Drawing for the job (mm, zero at the part's lowest x, y, z). A direction names the side the tool comes from. Coordinates: 2 decimals unless noted, no trailing zeros. Order: outer loops, then holes, each group sorted by start corner. A loop starts at its lowest first (then second) coordinate and runs counter-clockwise, first axis right, second up.
1) Tool access for the marked faces 1 and 2: list every direction of +Z, -Z, +X, -X, +Y, -Y with a clear straight run to the whole face (end or side of a thin tool).
2) Cut at B-B (z = 39). List the corners of the cut face in (x, y).
3) Pin check, flat tips, straight feed: pin 1 Ø1.5 at (y, z) = (34.5, 56.5) entering from +X; pin 2 Ø2 at (x, y) = (11.5, 38.5) entering from +Z; pin 3 Ø1.5 at (y, z) = (15.5, 17.5) entering from -X. Stop position of each tip, or through.
4) Wall check: L1, parallel to Y at x = 68.5, z = 47.5; L2, parallel to Z at x = 66.5, y = 35.5; L3, parallel to Z at x = 43.5, y = 28. Give the ranges that are in metal, low to high.
5) Cut at A-A (x = 54). List the corners of the cut face in (y, z), and give its area (3 significant figures).
6) Mould opens along Z. For the marked faces 3, 4 and 5 say: +Z half, -Z half, draft (parallel to the pull), parting line (faces both ways), or undercut.
7) Cut at D-D (x = 7). List the corners of the cut face in (y, z).
8) Cut at C-C (y = 46). List the corners of the cut face in (x, z).
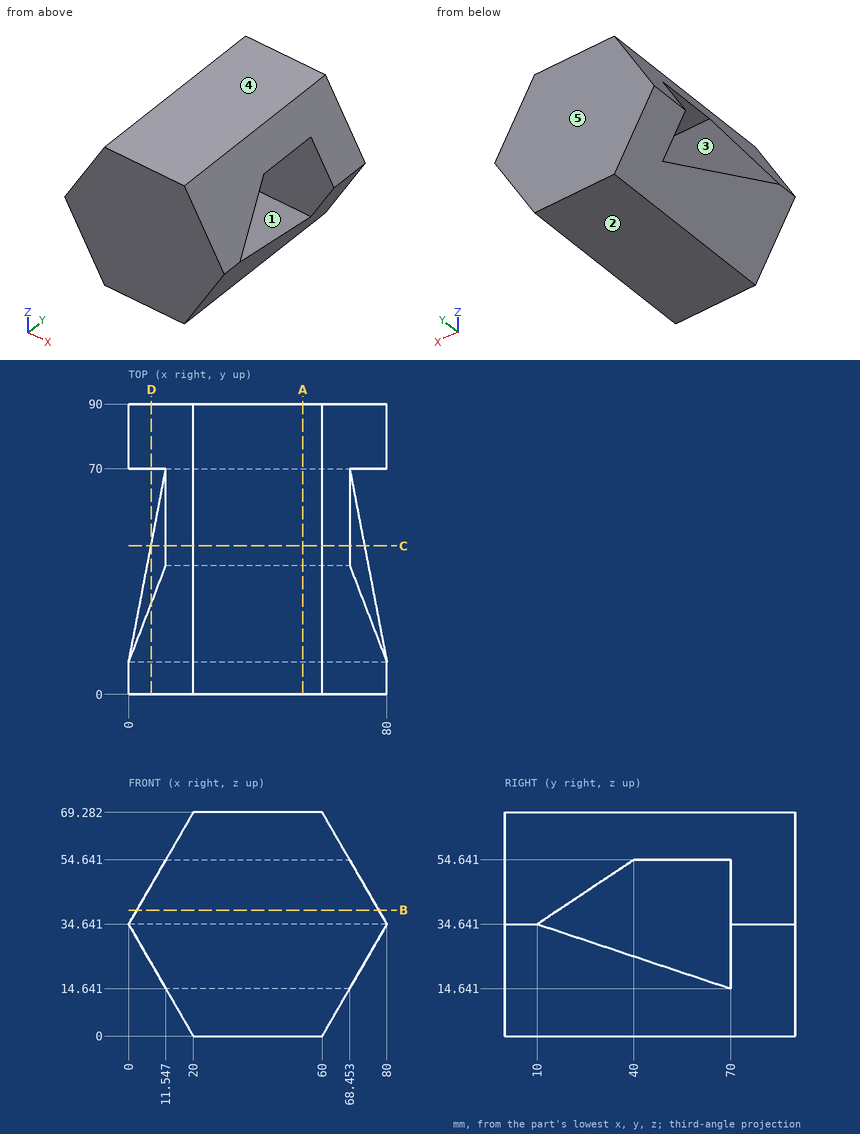
Geometry check:
1. face 1: +X, -X
1. face 2: -Z, +X, -X, +Y, -Y
2. outline: (2.52, 0) - (77.48, 0) - (77.48, 16.54) - (2.52, 16.54) - close; (2.52, 70) - (77.48, 70) - (77.48, 90) - (2.52, 90) - close
3. pin 1: stops at x = 67.81
3. pin 2: stops at z = 56.29
3. pin 3: stops at x = 9.46
4. L1: y = 0 to 29.29, 70 to 90
4. L2: z = 11.26 to 26.14, 51.64 to 58.02
4. L3: z = 0 to 28.64, 46.64 to 69.28
5. outline: (0, 0) - (90, 0) - (90, 69.28) - (0, 69.28) - close; hole (10, 34.64) - (70, 14.64) - (70, 54.64) - (40, 54.64) - close
5. area: 4,740 mm2
6. face 3: undercut
6. face 4: +Z half
6. face 5: draft
7. outline: (0, 22.52) - (46.37, 22.52) - (10, 34.64) - (28.19, 46.77) - (0, 46.77) - close; (70, 22.52) - (90, 22.52) - (90, 46.77) - (70, 46.77) - close
8. outline: (6.93, 22.64) - (20, 0) - (60, 0) - (73.07, 22.64) - close; (11.55, 54.64) - (68.45, 54.64) - (60, 69.28) - (20, 69.28) - close
